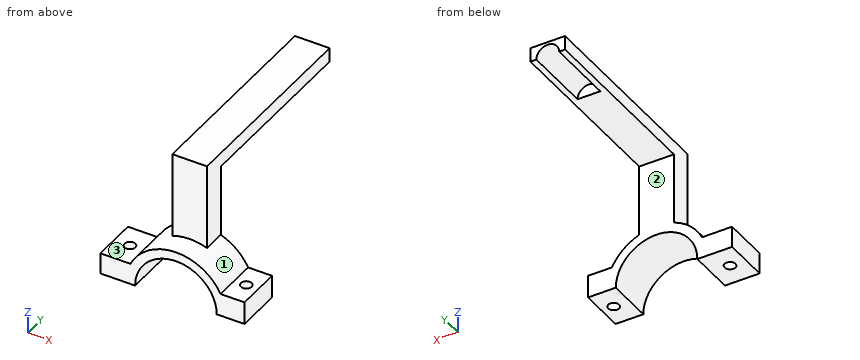
from build123d import *

# Parameters (mm, degrees)
SKETCH_1_R             = 17.63
SKETCH_1_R_2           = 14.34
EXTRUDE_1_DEPTH        = 16.05
EXTRUDE_1_2_DEPTH      = 9.77
EXTRUDE_1_2_DEPTH_BACK = 3
SKETCH_2_W             = 16
SKETCH_2_H             = 16.05
SKETCH_3_W             = 3.41
SKETCH_3_H             = 16
CUT_EXTRUDE_1_DEPTH    = 37.411121927
SKETCH_4_R             = 1.91
CUT_EXTRUDE_2_DEPTH    = 39.675463798
EXTRUDE_2_DEPTH        = 4
EXTRUDE_2_DEPTH_BACK   = 2.77
SKETCH_5_W             = 12.19
SKETCH_5_H             = 8.263625949
SKETCH_6_W             = 12.19
SKETCH_6_H             = 6.77
EXTRUDE_3_DEPTH        = 63
SKETCH_8_W             = 12.19
SKETCH_8_H             = 6.77
EXTRUDE_4_DEPTH        = 0.16
EXTRUDE_5_DEPTH        = 3.16
EXTRUDE_5_DEPTH_BACK   = 10
SKETCH_12_W            = 16
SKETCH_12_H            = 16.05
SKETCH_13_W            = 1.21
SKETCH_13_H            = 16
CUT_EXTRUDE_3_DEPTH    = 73.543164889
SKETCH_14_R            = 1.91
CUT_EXTRUDE_4_DEPTH    = 90.07387176
SKETCH_15_R            = 4.05
CUT_EXTRUDE_5_DEPTH    = 24
SKETCH_16_W            = 56.400519221
SKETCH_16_H            = 19.935010357
CUT_EXTRUDE_6_DEPTH    = 73.088971918
SKETCH_17_W            = 12.19
SKETCH_17_H            = 71.423625949
EXTRUDE_7_DEPTH        = 25
SKETCH_18_W            = 26.793372528
SKETCH_18_H            = 63.398625949
CUT_EXTRUDE_7_DEPTH    = 25
SKETCH_19_R            = 4
CUT_EXTRUDE_8_DEPTH    = 24


with BuildPart() as part:
    # 草圖1 → Extrude 1 (new body)
    with BuildSketch(Plane(origin=(0, 0, 0), x_dir=(1, 0, 0), z_dir=(0, 1, 0))):
        Circle(SKETCH_1_R)
        Circle(SKETCH_1_R_2, mode=Mode.SUBTRACT)
    extrude(amount=EXTRUDE_1_DEPTH)

    # 草圖2 → Extrude 1 2 (add, two sides: drawn at the far end of the back side and taken through both)
    with BuildSketch(Plane(origin=(17.75, 0, 0), x_dir=(0, 0, -1), z_dir=(1, 0, 0)).offset(-EXTRUDE_1_2_DEPTH_BACK)):
        with Locations((0, 8.025)):
            Rectangle(SKETCH_2_W, SKETCH_2_H)
    extrude(amount=EXTRUDE_1_2_DEPTH + EXTRUDE_1_2_DEPTH_BACK)

    # 草圖3 → 除料-伸長1 (cut, through all)
    with BuildSketch(Plane(origin=(0, 16.05, 0), x_dir=(1, 0, 0), z_dir=(0, 1, 0))):
        with Locations((25.815, 0)):
            Rectangle(SKETCH_3_W, SKETCH_3_H)
    extrude(amount=-CUT_EXTRUDE_1_DEPTH, mode=Mode.SUBTRACT)

    # 草圖4 → 除料-伸長2 (cut, through all)
    with BuildSketch(Plane.XY.offset(8)):
        with Locations((19.910203689, 8.025)):
            Circle(SKETCH_4_R)
    extrude(amount=-CUT_EXTRUDE_2_DEPTH, mode=Mode.SUBTRACT)

    # 草圖5 → 填料-伸長2 (add, two sides: drawn at the far end of the back side and taken through both)
    with BuildSketch(Plane.XY.offset(17.75).offset(-EXTRUDE_2_DEPTH_BACK)):
        with Locations((0, 12.156812974)):
            Rectangle(SKETCH_5_W, SKETCH_5_H)
    extrude(amount=EXTRUDE_2_DEPTH + EXTRUDE_2_DEPTH_BACK)

    # 草圖6 → 填料-伸長3 (add)
    with BuildSketch(Plane(origin=(0, 16.288625949, 0), x_dir=(1, 0, 0), z_dir=(0, 1, 0))):
        with Locations((0, -18.365)):
            Rectangle(SKETCH_6_W, SKETCH_6_H)
    extrude(amount=EXTRUDE_3_DEPTH)

    # 草圖8 → 填料-伸長4 (add)
    with BuildSketch(Plane(origin=(0, 79.288625949, 0), x_dir=(1, 0, 0), z_dir=(0, 1, 0))):
        with Locations((0, -18.365)):
            Rectangle(SKETCH_8_W, SKETCH_8_H)
    extrude(amount=EXTRUDE_4_DEPTH)

    # 草圖12 → 填料-伸長5 (add, two sides: drawn at the far end of the back side and taken through both)
    with BuildSketch(Plane(origin=(-17.75, 0, 0), x_dir=(0, 0, -1), z_dir=(1, 0, 0)).offset(-EXTRUDE_5_DEPTH_BACK)):
        with Locations((0.543544944, 8.025)):
            Rectangle(SKETCH_12_W, SKETCH_12_H)
    extrude(amount=EXTRUDE_5_DEPTH + EXTRUDE_5_DEPTH_BACK)

    # 草圖13 → 除料-伸長3 (cut, through all)
    with BuildSketch(Plane(origin=(0, 16.05, 0), x_dir=(1, 0, 0), z_dir=(0, 1, 0))):
        with Locations((-27.145, 0.543544944)):
            Rectangle(SKETCH_13_W, SKETCH_13_H)
    extrude(amount=-CUT_EXTRUDE_3_DEPTH, mode=Mode.SUBTRACT)

    # 草圖14 → 除料-伸長4 (cut, through all)
    with BuildSketch(Plane(origin=(0, 0, -8.543544944), x_dir=(-1, 0, 0), z_dir=(0, 0, -1))):
        with Locations(Location((20.980783679, 8.025, 0), (0, 0, 90))):
            Circle(SKETCH_14_R)
    extrude(amount=-CUT_EXTRUDE_4_DEPTH, mode=Mode.SUBTRACT)

    # 草圖15 → 除料-伸長5 (cut)
    with BuildSketch(Plane(origin=(0, 79.448625949, 0), x_dir=(1, 0, 0), z_dir=(0, 1, 0))):
        with Locations((0, -14.98)):
            Circle(SKETCH_15_R)
    extrude(amount=-CUT_EXTRUDE_5_DEPTH, mode=Mode.SUBTRACT)

    # 草圖16 → 除料-伸長6 (cut, through all)
    with BuildSketch(Plane(origin=(0, 16.05, 0), x_dir=(1, 0, 0), z_dir=(0, 1, 0))):
        with Locations((-4.090259611, 9.967505179)):
            Rectangle(SKETCH_16_W, SKETCH_16_H)
    extrude(amount=-CUT_EXTRUDE_6_DEPTH, mode=Mode.SUBTRACT)

    # 草圖17 → 填料-伸長7 (add)
    with BuildSketch(Plane.XY.offset(21.75)):
        with Locations((0, 43.736812975)):
            Rectangle(SKETCH_17_W, SKETCH_17_H)
    extrude(amount=EXTRUDE_7_DEPTH)

    # 草圖18 → 除料-伸長7 (cut)
    with BuildSketch(Plane.ZY.offset(6.095)):
        with Locations((28.376686264, 47.749312975)):
            Rectangle(SKETCH_18_W, SKETCH_18_H)
    extrude(amount=-CUT_EXTRUDE_7_DEPTH, mode=Mode.SUBTRACT)

    # 草圖19 → 除料-伸長8 (cut)
    with BuildSketch(Plane(origin=(0, 79.448625949, 0), x_dir=(1, 0, 0), z_dir=(0, 1, 0))):
        with Locations((0, -41.773372528)):
            Circle(SKETCH_19_R)
    extrude(amount=-CUT_EXTRUDE_8_DEPTH, mode=Mode.SUBTRACT)


solid = part.part
Build history of the part. All positions in model axes, mm. Face numbers are marked on the shaded views. A direction names the side the tool comes from. Give positions to 0.01 mm unless a question says otherwise; leave off trailing zeros. Order: outer loops, then holes, each group sorted by start corner. A loop starts at its lowest first (then second) coordinate and runs counter-clockwise, first axis right, second up. Notation, with made-up numbers: M 2,32.5 L 26,32.5 A20 cw 26,40.5 Z; hole C -3,48 d4. An arc over 180 degrees is marked long. Use one line per item in the form item = value.
1) Saw through at B-B (y = 73.5). Give the cut face in (x, z) (3 decimals).
Calculated:
outline = M -6.095,41.773 L -4,41.773 A4 cw 4,41.773 L 6.095,41.773 L 6.095,46.75 L -6.095,46.75 Z
2) Saw through at C-C (z = 24). Give the cut face in (x, y) (3 decimals).
Calculated:
outline = M -6.095,8.025 L 6.095,8.025 L 6.095,16.05 L -6.095,16.05 Z
3) Tool access for the marked faces 1, 2 and 3: list every direction of +Z, -Z, +X, -X, +Y, -Y with a clear straight run to the whole face (end or side of a thin tool).
Calculated:
face_1 = +Z, -Y
face_2 = -Z, +X, -X, +Y
face_3 = +Z, -X, +Y, -Y
4) Saw through at D-D (y = 49). Give the cut face in (x, z) (3 decimals), plus the area to 3 significant figures.
Calculated:
outline = M -6.095,41.773 L 6.095,41.773 L 6.095,46.75 L -6.095,46.75 Z
area = 60.7 mm2
5) Saw through at A-A (x = 0). Give the cut face in (y, z) (3 decimals).
Calculated:
outline = M 0,14.34 L 16.05,14.34 L 16.05,41.773 L 55.449,41.773 L 55.449,45.773 L 79.449,45.773 L 79.449,46.75 L 8.025,46.75 L 8.025,17.63 L 0,17.63 Z
6) Drop flat-ended pins along their axis: pin 1 (15 mm diameter, centred on y = 40, z = 39, fed in from -X) (3 decimals); pin 2 (8.5 mm diameter, centred on x = -23, y = 4, fed in from +Z); pin 3 (13.5 mm diameter, centred on x = 1.5, y = 35, fed in from -Z); pin 4 (4 mm diameter, centred on x = -10.5, z = 12.5, fed in from -Y). Give the stop position or say it passes through.
Calculated:
pin_1 = -6.095
pin_2 = 7.46
pin_3 = 41.77
pin_4 = 0
7) Probe probe 1 along X at (y, z) = (19.5, 45) (3 decimals); probe 2 along Z at (x, y) = (-23.5, 7.5); probe 3 along Z at (x, y) = (2, 18). List the from-to ranges inside material, lowest first.
Calculated:
probe_1 = -6.095 to 6.095
probe_2 = 0 to 7.46
probe_3 = 41.77 to 46.75
